Model file for the job. Use its own axes, mm. A direction names the side the tool comes from. Round coordinates to 2 decimals unless told otherwise and drop trailing zeros. Loops run counter-clockwise (first coordinate to the right, second up) from the corner with the lowest first, then second, coordinate; pieces in that order, holes last. Notation, with made-up numbers: (40.5, -9) - (61.5, -9) arc R26 ccw to (61.5, 7) - close; hole circle Ø6 at (37, 69). An arc over 180 degrees is marked (long way). Use one line per item in the form item = value.
from build123d import *

# Parameters (mm, degrees)
SKETCH1_W               = 350
SKETCH1_H               = 30
BOSS_EXTRUDE1_DEPTH     = 15
CUT_EXTRUDE2_DEPTH      = 353.562051276
CUT_EXTRUDE2_DEPTH_BACK = 353.562051276
SKETCH3_R               = 5
FILLET3_R               = 15
CUT_EXTRUDE3_DEPTH      = 353.562051276
CUT_EXTRUDE3_DEPTH_BACK = 10
SKETCH4_R               = 5
FILLET4_R               = 5
CUT_EXTRUDE4_REACH      = 353.603
SKETCH6_W               = 245
SKETCH6_H               = 5
FILLET6_R               = 5


with BuildPart() as part:
    # Sketch1 → Boss-Extrude1 (new, symmetric)
    with BuildSketch(Plane.XY):
        with Locations((175, 15)):
            Rectangle(SKETCH1_W, SKETCH1_H)
    extrude(amount=BOSS_EXTRUDE1_DEPTH, both=True)

    # Sketch3 → Cut-Extrude2 (cut, two sides: drawn at the far end of the back side and taken through both)
    with BuildSketch(Plane.XY.offset(15).offset(-CUT_EXTRUDE2_DEPTH_BACK)):
        with Locations((15, 15)):
            Circle(SKETCH3_R)
        with Locations((335, 15)):
            Circle(SKETCH3_R)
    extrude(amount=CUT_EXTRUDE2_DEPTH + CUT_EXTRUDE2_DEPTH_BACK, mode=Mode.SUBTRACT)

    # Fillet3
    fillet3_edges = [part.edges().sort_by_distance(p)[0] for p in [
        (350, 0, 0),
        (350, 30, 0),
        (0, 0, 0),
        (0, 30, 0),
    ]]
    fillet(fillet3_edges, radius=FILLET3_R - 0.0001)  # a hair under: the kernel refuses the full size

    # Sketch4 → Cut-Extrude3 (cut, two sides: drawn at the far end of the back side and taken through both)
    with BuildSketch(Plane.XY.offset(15).offset(-CUT_EXTRUDE3_DEPTH_BACK)):
        with BuildLine():
            Line((130, 30), (130, 0))
            Line((130, 0), (335.0001, 0))
            ThreePointArc((335.0001, 0), (345.606631007, 4.393368993), (350, 14.9999))
            Line((350, 14.9999), (350, 15.0001))
            ThreePointArc((350, 15.0001), (345.606631007, 25.606631007), (335.0001, 30))
            Line((335.0001, 30), (130, 30))
        make_face()
        with Locations((335, 15)):
            Circle(SKETCH4_R, mode=Mode.SUBTRACT)
    extrude(amount=CUT_EXTRUDE3_DEPTH + CUT_EXTRUDE3_DEPTH_BACK, mode=Mode.SUBTRACT)

    # Fillet4
    fillet4_edges = [part.edges().sort_by_distance(p)[0] for p in [
        (130, 15, 15),
    ]]
    fillet(fillet4_edges, radius=FILLET4_R)

    # Sketch6 → Cut-Extrude4 (cut, up to next)
    with BuildSketch(Plane.XZ, mode=Mode.PRIVATE) as cut_extrude4_sk1:
        with Locations((252.5, 2.5)):
            Rectangle(SKETCH6_W, SKETCH6_H)
    cut_extrude4_tool1 = extrude(cut_extrude4_sk1.sketch, amount=-CUT_EXTRUDE4_REACH, mode=Mode.PRIVATE) & part.part
    add(cut_extrude4_tool1.solids().sort_by_distance((252.5, 0, 2.5))[0], mode=Mode.SUBTRACT)

    # Fillet6
    fillet6_edges = [part.edges().sort_by_distance(p)[0] for p in [
        (130, 15, 0),
    ]]
    fillet(fillet6_edges, radius=FILLET6_R)


solid = part.part
1. Wall check: probe 1 along X at (y, z) = (15, -8); probe 2 along Y at (x, z) = (335, -8.75); probe 3 along Z at (x, y) = (235, 26). Give the ranges that are in metal, low to high.
Geometry check:
probe_1 = 0 to 10, 20 to 330, 340 to 350
probe_2 = 0 to 10, 20 to 30
probe_3 = -15 to 0
2. Cut at B-B, the plane x = 201. Give the cut face in (y, z).
Geometry check:
outline = (0, -15) - (30, -15) - (30, 0) - (0, 0) - close
3. Tool access for faces 4 (the cylindrical face through (345.49, 4.28, -7.4)), 5 (the flat face through (241, 15, 0)): list every direction of +Z, -Z, +X, -X, +Y, -Y with a clear straight run to the whole face (end or side of a thin tool).
Geometry check:
face_4 = +Z, -Z, +X, -Y
face_5 = +Z, +X, +Y, -Y
4. Flat gauge pins, fed straight in: pin 1 (1.5 mm diameter, centred on y = 20.5, z = 6.5, fed in from +X); pin 2 (1.5 mm diameter, centred on y = 4, z = 2.5, fed in from -X); pin 3 (13 mm diameter, centred on x = 335, y = 15, fed in from -Z); pin 4 (6 mm diameter, centred on x = 151, y = 27, fed in from +Z). Where does each tip first touch, or does it go through?
Geometry check:
pin_1 = 130
pin_2 = 4.05
pin_3 = -15
pin_4 = 0
5. Cut at A-A, the plane z = -6. Give the number of separate pieces and of enclosed holes in the cut face, plus the area to 3 significant figures.
Geometry check:
separate_pieces = 1
enclosed_holes = 2
area = 10,100 mm^2
6. Pull direction X, two halves, no side cores. Call faces 1 (the cylindrical face through (339.619, 13.085, -7.605)), 2 (the cylindrical face through (345.49, 25.72, -7.6)), 3 (the cylindrical face through (4.28, 25.49, -0.21)): +X half, -X half, draft (parallel to the pull), parting line (faces both ways), or undercut.
Geometry check:
face_1 = undercut
face_2 = +X half
face_3 = -X half
